from build123d import *

# Parameters (mm, degrees)
CROQUIS1_R = 13.7


with BuildPart() as part:
    # Barrer1: sweep along a curve in space
    with BuildLine() as barrer1_path:
        Line((0, 0, 0), (-535, 0, 0))
        ThreePointArc((-535, 0, 0), (-545.606601718, 4.393398282, 0), (-550, 15, 0))
        Line((-550, 15, 0), (-550, 85, 0))
        Line((-550, 85, 0), (-550, 85, 30))
        Line((-550, 85, 30), (-550, 155, 30))
        ThreePointArc((-550, 155, 30), (-554.393398282, 165.606601718, 30), (-565, 170, 30))
        Line((-565, 170, 30), (-1000, 170, 30))
    # Croquis1 → Barrer1 (sweep)
    with BuildSketch(Plane(origin=(0, 0, 0), x_dir=(0, 0, -1), z_dir=(1, 0, 0))):
        Circle(CROQUIS1_R)
    sweep(path=barrer1_path.line, transition=Transition.RIGHT)


solid = part.part
CAD build for the part. Positions are in the model's coordinates, mm. A direction names the side the tool comes from. Round coordinates to 2 decimals unless told otherwise and drop trailing zeros. Write each loop counter-clockwise with the first axis right and the second up, starting at its lowest first coordinate (ties: lowest second). Pieces come first, ordered by that corner, then holes.
(1) 3-axis set-ups, long thin cutter, end or side, ignore diameter. For faces 1 (the face through (-785.545, 183.374, 32.97)), 2 (the face through (0, 0, 0)), 3 (the face through (-550.602, 123.036, 43.687)): which of +Z, -Z, +X, -X, +Y, -Y reach the whole face in a straight line?
(2) Drop flat-ended pins along their axis: P1, Ø1.5, axis at y = 148.5, z = 34.5, coming from the +X side; P2, Ø1.5, axis at y = 58, z = 10.5, coming from the -X side; P3, Ø8, axis at x = -397.5, z = 9.5, coming from the +Y side. Give the stop position or say it passes through.
(3) Probe line 1 along X through (y, z) = (86.5, 27); line 2 along X through (y, z) = (5.5, -7); line 3 along Y through (x, z) = (-706, 22.5). List the from-to ranges inside material, lowest first.
(4) Slice it at A-A, the plane z = 30. Write the cut outline in (x, y), and give its area (3 significant figures).
(5) Mould opens along Y. For faces 4 (the face through (-544.753, 48.136, -12.655)), 5 (the face through (-271.245, -9.259, 10.097)), 6 (the face through (-1000, 170, 30)) say: pulls with the +Y half, pulls with the -Y half, needs draft (parallel to the pull), parting line crosses it, or undercut.
(6) Slice it at C-C, the plane x = -836.5. Write the cut outline in (y, z).
(7) Slice it at B-B, the plane y = 107. Write the cut outline in (x, z), and give its area (3 significant figures).
From the geometry:
1. face 1: -X
1. face 2: +Z, -Z, +X, +Y, -Y
1. face 3: none
2. P1: stops at x = -536.82
2. P2: stops at x = -559.62
2. P3: stops at y = 12.55
3. line 1: x = -563.62 to -536.38
3. line 2: x = -560.03 to 0
3. line 3: y = 158.54 to 181.46
4. outline: (-1000, 156.3) - (-565, 156.3) arc R1.3 cw to (-563.7, 155) - (-563.7, 85) arc R13.7 ccw to (-536.3, 85) - (-536.3, 155) arc R28.7 ccw to (-565, 183.7) - (-1000, 183.7) - close
4. area: 14,800 mm2
5. face 4: undercut
5. face 5: parting line crosses it
5. face 6: needs draft
6. outline: circle Ø27.4 at (170, 30)
7. outline: circle Ø27.4 at (-550, 30)
7. area: 590 mm2
